The listing builds one solid part. Answer for the finished solid, in the listing's coordinates (mm). Face numbers are marked on the shaded views. A direction names the side the tool comes from. Round coordinates to 2 decimals unless told otherwise and drop trailing zeros. Write each loop counter-clockwise with the first axis right and the second up, starting at its lowest first coordinate (ties: lowest second). Pieces come first, ordered by that corner, then holes.
Item 1: Find section A-A on y = -14. Give the vertices of the cut face in (x, z), then the cut area to 3 significant figures.
Item 2: Find section D-D on z = 37. Give the vertices of the cut face in (x, y), then the cut area to 3 significant figures.
Item 3: Find section C-C on x = 72.5. Give the vertices of the cut face in (y, z).
Item 4: Each of these flat-tipped pins is pushed along its axis until it touches: pin 1 (10 mm diameter, centred on y = -28.5, z = 45.5, fed in from +X); pin 2 (6.5 mm diameter, centred on y = -16.5, z = 40.5, fed in from -X); pin 3 (6 mm diameter, centred on y = -24, z = 47.5, fed in from -X). Where does it stop, or does it pass through?
Item 5: Find the intervals of material crossed by probe 1 along Z at (x, y) = (-37.5, -11.5); probe 2 along Z at (x, y) = (-63, -15); probe 3 along Y at (x, z) = (-72, -7.5), in increasing order.
Item 6: Find section B-B on z = -6.5. Give the vertices of the cut face in (x, y).
Item 7: For a pull along Z with two mould halves and no side action, classify the marked faces 5, 6 and 7 as +Z half, -Z half, draft (parallel to the pull), parting line (faces both ways), or undercut.
Item 8: A tool of negligible diameter and unlimited length cuts with its end or side. For the marked faces 1, 2, 3 and 4, from which of +Z, -Z, +X, -X, +Y, -Y can it reach the whole face along a straight path? Write none if from no direction.
```python
from build123d import *

# Parameters (mm, degrees)
F0_W     = 190
F0_H     = 100
F1_DEPTH = 10
F3_DEPTH = 25
F4_DEPTH = 25


with BuildPart() as f1:
    # F0 (on Front) → F1 (new body)
    with BuildSketch(Plane.XZ):
        Rectangle(F0_W, F0_H)
    extrude(amount=F1_DEPTH)

    # F2 (on face) → F3 (join)
    with BuildSketch(Plane.XZ.offset(10)):
        Polygon((-49.491931, 40.968843), (-49.491931, 50), (-54.094203, 50), (-54.094203, 42.272657), (-95, 22.963328), (-95, 8.291027), (74.74266, -50), (76.602353, -47.408584), (-91.554888, 10.337997), (-91.554888, 21.052278), (-88.564485, 22.468217), align=None)
        Polygon((-30.388942, 50), (-33.300221, 50), (-33.300221, 40.968843), (-33.300221, 28.898658), (-61.637774, 18.919959), (-65.695935, 17.490931), (85.04647, -30.56908), (87.651487, -27.179441), (-54.094203, 18.012218), (-30.388942, 25.933994), align=None)
    extrude(amount=F3_DEPTH)

    # F2 (on face) → F4 (cut)
    with BuildSketch(Plane.XZ.offset(10)):
        Polygon((-57.566985, 10.273552), (-73.658094, 15.96733), (-75.863337, 11.080531), (-59.349135, 5.237044), align=None)
        Polygon((-7.86031, -4.662096), (-34.249816, 3.969805), (-36.453794, -2.258826), (-10.286281, -11.518101), align=None)
        Polygon((36.374753, -18.724323), (12.500672, -10.772827), (9.540769, -20.056697), (33.513222, -27.699645), align=None)
        Polygon((80.424149, -33.161463), (55.549646, -24.682663), (51.817555, -36.388537), (76.602353, -44.290479), align=None)
    extrude(amount=-F4_DEPTH, mode=Mode.SUBTRACT)


solid = f1.part
```
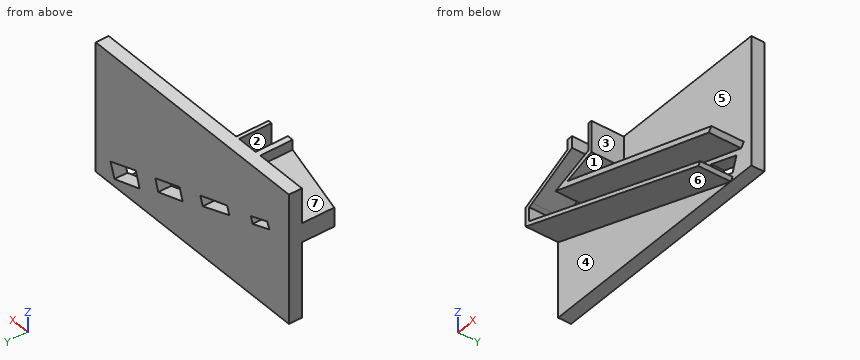
Check values:
1. outline: (-95, 8.29) - (74.74, -50) - (76.6, -47.41) - (-91.55, 10.34) - (-91.55, 21.05) - (-88.56, 22.47) - (-49.49, 40.97) - (-49.49, 50) - (-54.09, 50) - (-54.09, 42.27) - (-95, 22.96) - close; (-65.7, 17.49) - (85.05, -30.57) - (87.65, -27.18) - (-54.09, 18.01) - (-30.39, 25.93) - (-30.39, 50) - (-33.3, 50) - (-33.3, 28.9) - close
1. area: 1,560 mm2
2. outline: (-95, -10) - (-65.26, -10) - (-65.26, -35) - (-57.87, -35) - (-57.87, -10) - (-33.3, -10) - (-33.3, -35) - (-30.39, -35) - (-30.39, -10) - (95, -10) - (95, 0) - (-95, 0) - close
2. area: 2,160 mm2
3. outline: (-35, -49.23) - (-10, -49.23) - (-10, -50) - (0, -50) - (0, -42.98) - (-10, -42.98) - (-10, -46) - (-35, -46) - close; (-35, -26.57) - (-10, -26.57) - (-10, -30.46) - (0, -30.46) - (0, 50) - (-10, 50) - (-10, -22.35) - (-35, -22.35) - close
4. pin 1: stops at x = -30.39
4. pin 2: stops at x = -64.73
4. pin 3: stops at x = -54.09
5. probe 1: z = -11.45 to -8.22, 8.5 to 12.72, 23.56 to 27.42
5. probe 2: z = -2.7 to 0.53, 16.63 to 18.44, 34.57 to 38.07
5. probe 3: y = -10 to 0
6. outline: (-95, -10) - (-51.93, -10) - (-51.93, -35) - (-42.52, -35) - (-42.52, -10) - (-24.47, -10) - (-24.47, 0) - (-95, 0) - close; (-8.51, -10) - (9.55, -10) - (9.55, -35) - (22.79, -35) - (22.79, -10) - (95, -10) - (95, 0) - (-8.51, 0) - close
7. face 5: undercut
7. face 6: -Z half
7. face 7: +Z half
8. face 1: +X, -Y
8. face 2: +Z, -Y
8. face 3: +Z, +X, -Y
8. face 4: -Z, -X, -Y
